from build123d import *

# Parameters (mm, degrees)
F0_W     = 240
F0_H     = 100
F0_R     = 8
F1_DEPTH = 3
F2_R     = 10


with BuildPart() as f1:
    # F0 (on Front) → F1 (new body)
    with BuildSketch(Plane.XZ):
        Rectangle(F0_W, F0_H)
        with Locations((0, -30)):
            Circle(F0_R, mode=Mode.SUBTRACT)
        Circle(F0_R, mode=Mode.SUBTRACT)
        with Locations((0, 30)):
            Circle(F0_R, mode=Mode.SUBTRACT)
    extrude(amount=F1_DEPTH)

    # F2
    f2_edges = [f1.edges().sort_by_distance(p)[0] for p in [
        (-120, -1.5, 50),
        (-120, -1.5, -50),
        (120, -1.5, 50),
        (120, -1.5, -50),
    ]]
    fillet(f2_edges, radius=F2_R)


solid = f1.part
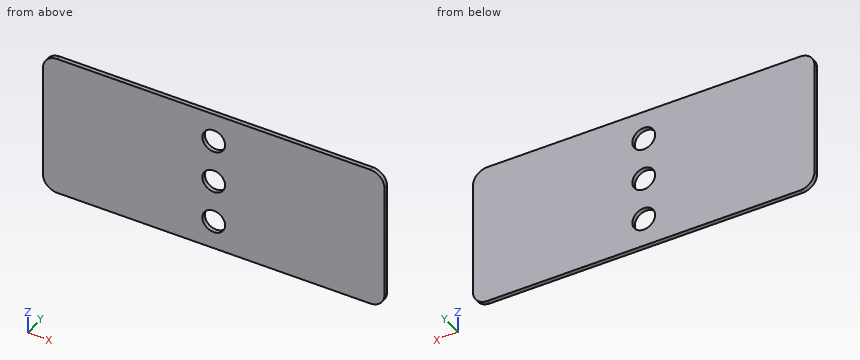
Geometry check sheet. Reference: the model listing, model coordinates, mm. Give positions to 0.01 mm unless a question says otherwise; leave off trailing zeros. Order: outer loops, then holes, each group sorted by start corner. A loop starts at its lowest first (then second) coordinate and runs counter-clockwise, first axis right, second up.
1. Sectioned sample at B-B (y = -0.7). Record the boundary of the cut face in (x, z).
Completed:
outline: (-120, -40) arc R10 ccw to (-110, -50) - (110, -50) arc R10 ccw to (120, -40) - (120, 40) arc R10 ccw to (110, 50) - (-110, 50) arc R10 ccw to (-120, 40) - close; hole circle Ø16 at (0, -30); hole circle Ø16 at (0, 0); hole circle Ø16 at (0, 30)
2. Sectioned sample at A-A (z = -30). Record the boundary of the cut face in (x, y).
Completed:
outline: (-120, -3) - (-8, -3) - (-8, 0) - (-120, 0) - close; (8, -3) - (120, -3) - (120, 0) - (8, 0) - close
3. Scan lines: line 1 (Z direction, x = 0, y = -1.6); line 2 (X direction, y = -1.5, z = -7); line 3 (X direction, y = -0.7, z = 31). Record each from-to range of solid material in increasing order.
Completed:
line 1: z = -50 to -38, -22 to -8, 8 to 22, 38 to 50
line 2: x = -120 to -3.87, 3.87 to 120
line 3: x = -120 to -7.94, 7.94 to 120
4. Sectioned sample at C-C (z = -3). Record the boundary of the cut face in (x, y), then the cut area to 3 significant figures.
Completed:
outline: (-120, -3) - (-7.42, -3) - (-7.42, 0) - (-120, 0) - close; (7.42, -3) - (120, -3) - (120, 0) - (7.42, 0) - close
area: 676 mm2
